from build123d import *

# Parameters (mm, degrees)
BOSS_EXTRUDE1_DEPTH  = 10
BOSS_EXTRUDE2_DEPTH  = 70
SKETCH1_6_W          = 28.50000000000001
SKETCH1_6_H          = 10
CUT_EXTRUDE1_DEPTH   = 80
SKETCH1_7_W          = 28.50000000000001
SKETCH1_7_H          = 10
BOSS_EXTRUDE4_DEPTH  = 30
SKETCH1_8_R          = 2.0000000000000004
SKETCH1_8_R_2        = 1.9999999999999967
CUT_EXTRUDE2_DEPTH   = 30
SKETCH1_9_R          = 4.000000000000002
SKETCH1_9_R_2        = 4.000000000000007
CUT_EXTRUDE3_DEPTH   = 4
SKETCH1_11_R         = 32.50000000000001
SKETCH1_11_R_2       = 25.499999999999993
BOSS_EXTRUDE6_DEPTH  = 20
FILLET1_R            = 10
SKETCH1_12_R         = 4.000000000000005
BOSS_EXTRUDE7_DEPTH  = 19
BOSS_EXTRUDE13_DEPTH = 70
BOSS_EXTRUDE17_DEPTH = 40
CUT_EXTRUDE4_DEPTH   = 40
CUT_EXTRUDE5_DEPTH   = 3
FILLET2_R            = 5
FILLET3_R            = 2


# Read off the part's stored shape, not the designer's step: Boss-Extrude17
with BuildPart() as part:
    # Sketch1 → Boss-Extrude1 (new body)
    with BuildSketch(Plane.XY):
        Polygon((-10.000000000000002, 10.000000000000002), (90, 10.000000000000002), (90.00000000000003, -95), (-9.999999999999988, -95), align=None)
    extrude(amount=-BOSS_EXTRUDE1_DEPTH)

    # Sketch1_3 → Boss-Extrude2 (add)
    with BuildSketch(Plane.XY):
        Polygon((-10.000000000000002, 10.000000000000002), (90, 10.000000000000002), (90.00000000000003, -95), (-9.999999999999988, -95), align=None)
        Polygon((0, 0), (80, 0), (80.00000000000001, -85), (1.041e-14, -85), align=None, mode=Mode.SUBTRACT)
    extrude(amount=BOSS_EXTRUDE2_DEPTH)

    # Sketch1_6 → Cut-Extrude1 (cut)
    with BuildSketch(Plane.XY):
        with Locations((40.000000000000014, -90)):
            Rectangle(SKETCH1_6_W, SKETCH1_6_H)
    extrude(amount=CUT_EXTRUDE1_DEPTH, mode=Mode.SUBTRACT)

    # Sketch1_7 → Boss-Extrude4 (add)
    with BuildSketch(Plane.XY):
        with Locations((40.000000000000014, -90)):
            Rectangle(SKETCH1_7_W, SKETCH1_7_H)
    extrude(amount=BOSS_EXTRUDE4_DEPTH)

    # Sketch1_8 → Cut-Extrude2 (cut)
    with BuildSketch(Plane.XY):
        with Locations((6.000000000000001, -6)):
            Circle(SKETCH1_8_R)
        with Locations((74.00000000000001, -79)):
            Circle(SKETCH1_8_R_2)
    extrude(amount=-CUT_EXTRUDE2_DEPTH, mode=Mode.SUBTRACT)

    # Sketch1_9 → Cut-Extrude3 (cut)
    with BuildSketch(Plane.XY):
        with Locations((6.000000000000001, -6)):
            Circle(SKETCH1_9_R)
        with Locations((74.00000000000001, -79)):
            Circle(SKETCH1_9_R_2)
    extrude(amount=-CUT_EXTRUDE3_DEPTH, mode=Mode.SUBTRACT)

    # Sketch1_11 → Boss-Extrude6 (add)
    with BuildSketch(Plane.XY):
        with Locations((40.00000000000001, -37)):
            Circle(SKETCH1_11_R)
        with Locations((40.00000000000001, -37)):
            Circle(SKETCH1_11_R_2, mode=Mode.SUBTRACT)
    extrude(amount=BOSS_EXTRUDE6_DEPTH)

    # Fillet1
    fillet1_edges = [part.edges().sort_by_distance(p)[0] for p in [
        (54.25000000000002, -90, 30),
        (25.750000000000014, -90, 30),
    ]]
    fillet(fillet1_edges, radius=FILLET1_R)

    # Sketch1_12 → Boss-Extrude7 (add)
    with BuildSketch(Plane.XY):
        with Locations((40.00000000000001, -20.887152181723966)):
            Circle(SKETCH1_12_R)
    extrude(amount=BOSS_EXTRUDE7_DEPTH)

    # Sketch1_18 → Boss-Extrude13 (add)
    with BuildSketch(Plane.XY):
        with BuildLine():
            Line((54.25000000000002, -7.790626504493452), (54.25000000000002, 0))
            Line((54.25000000000002, 0), (25.750000000000014, 0))
            Line((25.750000000000014, 0), (25.750000000000014, -7.790626504494099))
            ThreePointArc((25.749999999999222, -7.7906265044938365), (39.999999999999574, -4.499999999999993), (54.25000000000003, -7.79062650449346))
        make_face()
    extrude(amount=BOSS_EXTRUDE13_DEPTH)

    # Boss-Extrude17 outline → Boss-Extrude17 (add)
    with BuildSketch(Plane.XY):
        with BuildLine():
            ThreePointArc((11.1, -44), (10.264331183, -37), (11.1, -30))
            Line((11.1, -30), (0, -30))
            Line((0, -30), (0, -44))
            Line((0, -44), (11.1, -44))
        make_face()
        with BuildLine():
            Line((80, -30), (68.9, -30))
            ThreePointArc((68.9, -30), (69.735668817, -37), (68.9, -44))
            Line((68.9, -44), (80, -44))
            Line((80, -44), (80, -30))
        make_face()
    extrude(amount=BOSS_EXTRUDE17_DEPTH)

    # Sketch1_25 → Cut-Extrude4 (cut)
    with BuildSketch(Plane.XY):
        with BuildLine():
            ThreePointArc((10.264331182904264, -36.99999999999999), (10.473987495649993, -40.52485256329489), (11.100000000000009, -44))
            Line((11.100000000000005, -44.00000000000001), (11.100000000000003, -37))
            Line((11.100000000000003, -37), (10.264331182904264, -37))
        make_face()
        with BuildLine():
            ThreePointArc((11.100000000000005, -30), (10.473987495649993, -33.47514743670511), (10.264331182904264, -36.99999999999999))
            Line((10.264331182904264, -37), (11.100000000000003, -37))
            Line((11.100000000000003, -37), (11.100000000000003, -30.00000000000001))
        make_face()
        with BuildLine():
            Line((68.90000000000002, -37), (68.90000000000002, -44))
            ThreePointArc((68.9, -44), (69.52601250435002, -40.52485256329488), (69.73566881709576, -37.00000000000001))
            Line((69.73566881709576, -37), (68.90000000000002, -37))
        make_face()
        with BuildLine():
            Line((68.90000000000002, -37), (69.73566881709576, -37))
            ThreePointArc((69.73566881709576, -37), (69.52601250435002, -33.475147436705115), (68.9, -30))
            Line((68.90000000000002, -30), (68.90000000000002, -37))
        make_face()
    extrude(amount=CUT_EXTRUDE4_DEPTH, mode=Mode.SUBTRACT)

    # Sketch2 → Cut-Extrude5 (cut)
    with BuildSketch(Plane(origin=(0, -85, 0), x_dir=(1, 0, 0), z_dir=(0, 1, 0))):
        with BuildLine():
            Line((60.57528408294713, -36.561798125074915), (62.8218137104663, -81.75240597499271))
            ThreePointArc((62.8218137104663, -81.75240597499271), (43.26937458327802, -103.35053501369867), (21.671245544572063, -83.7980958865104))
            Line((21.671245544572063, -83.7980958865104), (19.42471591705289, -38.6074880365926))
            ThreePointArc((19.42471591705289, -38.6074880365926), (38.977155044241165, -17.009358997886636), (60.57528408294713, -36.561798125074915))
        make_face()
    extrude(amount=-CUT_EXTRUDE5_DEPTH, mode=Mode.SUBTRACT)

    # Fillet2
    fillet2_edges = [part.edges().sort_by_distance(p)[0] for p in [
        (-10.000000000000002, 10.000000000000002, 30),
        (90, 10.000000000000002, 30),
        (90.00000000000003, -95, 30),
        (-9.999999999999988, -95, 30),
    ]]
    fillet(fillet2_edges, radius=FILLET2_R)

    # Fillet3
    fillet3_edges = [part.edges().sort_by_distance(p)[0] for p in [
        (14.500000000000014, -37.00000000000001, 20),
    ]]
    fillet(fillet3_edges, radius=FILLET3_R)


solid = part.part
Read the model definition and answer for the solid it produces. Units are mm, in the model's axes. A direction names the side the tool comes from. Round coordinates to 2 decimals unless told otherwise and drop trailing zeros. Order: outer loops, then holes, each group sorted by start corner. A loop starts at its lowest first (then second) coordinate and runs counter-clockwise, first axis right, second up. Notation, with made-up numbers: (43.25, -27.5) - (73.25, -27.5) arc R10 cw to (73.25, -15.5) - close; hole circle Ø5 at (20.25, -5). An arc over 180 degrees is marked (long way). Use one line per item in the form item = value. Start each with the question number.
(1) Flat-ended cylindrical pins translate along their axes: pin 1 Ø6.5 at (x, y) = (38.5, -21.5) entering from +Z; pin 2 Ø2 at (x, z) = (49, 57) entering from -Y; pin 3 Ø9 at (x, y) = (3, -36) entering from +Z; pin 4 Ø3.5 at (y, z) = (-92, 52.5) entering from +X. Find the tip coordinate at first contact, or state that the pin passes through.
(2) The part is cut by section D-D (y = -37). Give the vertices of the cut face in (x, z).
(3) For faces 4 (the face through (72, -80, -4)), 5 (the face through (41, -42, -10)), 6 (the face through (25.75, -92, 55)), determine the directions among +Z, -Z, +X, -X, +Y, -Y from which every point of the face is accessible in a straight line to the end or side of a thin tool.
(4) The part is cut by section B-B (y = -6). Give the vertices of the cut face in (x, z).
(5) The part is cut by section C-C (x = 40). Give the vertices of the cut face in (y, z), then the cut area to 3 significant figures.
(6) The part is cut by section A-A (x = 6). Give the vertices of the cut face in (y, z), then the cut area to 3 significant figures.
(7) Determine the mould class of faces 1 (the face through (25.75, -4, 35)), 2 (the face through (90, -42, 29)), 3 (the face through (-9, 8, 31)) for opening direction Y: +Y half, -Y half, draft (parallel to the pull), parting line (faces both ways), or undercut.
(8) Find the intervals of material crossed by line 1 along X through (y, z) = (-12, 57.5); line 2 along Y through (x, z) = (6, -7.55); line 3 along X through (y, z) = (-66.5, 8), in increasing order. Write a range as from..to.
Checked values:
q1.pin_1 = 19
q1.pin_2 = -6.08
q1.pin_3 = 70
q1.pin_4 = 89.99
q2.outline = (-10, -10) - (90, -10) - (90, 70) - (80, 70) - (80, 40) - (69.74, 40) - (69.74, 0) - (68.9, 0) - (68.9, 20) - (67.5, 20) arc R2 ccw to (65.5, 18) - (65.5, 0) - (14.5, 0) - (14.5, 18) arc R2 ccw to (12.5, 20) - (11.1, 20) - (11.1, 0) - (10.26, 0) - (10.26, 40) - (0, 40) - (0, 70) - (-10, 70) - close
q3.face_4 = +Z
q3.face_5 = -Z, +X, -X, +Y, -Y
q3.face_6 = +Z, -Y
q4.outline = (-10, -10) - (4, -10) - (4, -4) - (2, -4) - (2, 0) - (0, 0) - (0, 70) - (-10, 70) - close; (8, -10) - (90, -10) - (90, 70) - (80, 70) - (80, 0) - (54.25, 0) - (54.25, 70) - (49.76, 70) - (49.76, 20) - (30.24, 20) - (30.24, 70) - (25.75, 70) - (25.75, 0) - (10, 0) - (10, -4) - (8, -4) - close
q5.outline = (-95, -10) - (10, -10) - (10, 70) - (-4.5, 70) - (-4.5, 20) - (-9.5, 20) arc R2 ccw to (-11.5, 18) - (-11.5, 0) - (-16.89, 0) - (-16.89, 19) - (-24.89, 19) - (-24.89, 0) - (-62.5, 0) - (-62.5, 18) arc R2 ccw to (-64.5, 20) - (-69.5, 20) - (-69.5, 0) - (-85, 0) - (-85, 16.98) - (-88, 16.98) - (-88, 30) - (-95, 30) - close
q5.area = 2,760 mm^2
q6.outline = (-95, -10) - (-8, -10) - (-8, -4) - (-10, -4) - (-10, 0) - (-30, 0) - (-30, 40) - (-44, 40) - (-44, 0) - (-85, 0) - (-85, 70) - (-95, 70) - close; (-4, -10) - (10, -10) - (10, 70) - (0, 70) - (0, 0) - (-2, 0) - (-2, -4) - (-4, -4) - close
q6.area = 2,950 mm^2
q7.face_1 = undercut
q7.face_2 = draft
q7.face_3 = +Y half
q8.line_1 = -10..0, 80..90
q8.line_2 = -95..-8, -4..10
q8.line_3 = -10..0, 26.36..53.64, 80..90
